For this review, take the finished solid that the model builds, in its own axes (mm). Face numbers are marked on the shaded views. A direction names the side the tool comes from. Give positions to 0.01 mm unless a question says otherwise; leave off trailing zeros. Loops run counter-clockwise (first coordinate to the right, second up) from the corner with the lowest first, then second, coordinate; pieces in that order, holes last. Notation, with made-up numbers: (82, 13) -> (116, 13) arc R28 ccw to (116, 34) -> close; hole circle Ø4 at (7.5, 22.25). An arc over 180 degrees is marked (long way). One line per question, with ' | ' between items. Start each with the question number.
(1) Insertion check: P1, Ø12, axis at x = 32.5, z = -18, coming from the -Y side; P2, Ø5, axis at x = -20.5, y = -17.5, coming from the -Z side; P3, Ø3, axis at x = 11, y = -30.5, coming from the -Z side; P4, Ø2, axis at y = -15.5, z = 0, coming from the -X side. Each pin has a flat end and moves straight along its axis. Give the tip position at first contact, or say it passes through.
(2) Consider section A-A (y = -17.5). Write out the cut boundary in (x, z), and give its area (3 significant figures).
(3) Consider section C-C (x = 27). Write out the cut boundary in (y, z), and give its area (3 significant figures).
(4) Tool access review of the marked faces 1, 2 and 3: name each direction out of +Z, -Z, +X, -X, +Y, -Y from which nothing blocks a thin tool from reaching the whole face with its end or side.
(5) Draft analysis for pull direction X (two halves, no side actions). For the marked faces 4, 5 and 6, state which applies: +X half, -X half, draft (parallel to the pull), parting line (faces both ways), or undercut.
(6) Consider section D-D (y = -6.5). Write out the cut boundary in (x, z).
(7) Wall thickness on probe 1 along X at (y, z) = (-6, 5); probe 2 along Z at (x, y) = (22, -32.5); probe 3 along Y at (x, z) = (-35, 7): over which ranges is each line inside the solid? List them lowest first.
(8) Consider section B-B (z = 0). Write out the cut boundary in (x, y), and give its area (3 significant figures).
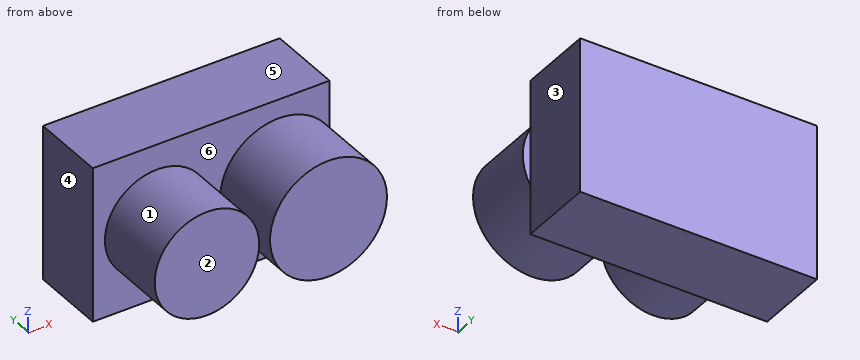
from build123d import *

# Parameters (mm, degrees)
F0_W     = 79.5864835382
F0_H     = 52.0435199142
F1_DEPTH = 12.7
F2_R     = 19.6570457416
F2_R_2   = 17.5585400789
F3_DEPTH = 25.4


with BuildPart() as f1:
    # F0 (on Front) → F1 (new body, symmetric)
    with BuildSketch(Plane.XZ):
        Rectangle(F0_W, F0_H)
    extrude(amount=F1_DEPTH, both=True)

    # F2 (on face) → F3 (join)
    with BuildSketch(Plane.XZ.offset(12.7)):
        with Locations((22.6829834282, 0)):
            Circle(F2_R)
        with Locations((-18.1834697723, 0)):
            Circle(F2_R_2)
    extrude(amount=F3_DEPTH)


solid = f1.part
A:
1) P1: stops at y = -38.1 | P2: stops at z = -17.56 | P3: stops at z = -16.81 | P4: stops at x = -35.74
2) outline: circle Ø35.12 at (-18.18, 0); circle Ø39.31 at (22.68, 0) | area: 2,180 mm^2
3) outline: (-38.1, -19.18) -> (-12.7, -19.18) -> (-12.7, -26.02) -> (12.7, -26.02) -> (12.7, 26.02) -> (-12.7, 26.02) -> (-12.7, 19.18) -> (-38.1, 19.18) -> close | area: 2,300 mm^2
4) face 1: -Y | face 2: +Z, -Z, +X, -X, -Y | face 3: +Z, -Z, +X, +Y
5) face 4: -X half | face 5: draft | face 6: undercut
6) outline: (-39.79, -26.02) -> (39.79, -26.02) -> (39.79, 26.02) -> (-39.79, 26.02) -> close
7) probe 1: x = -39.79 to 39.79 | probe 2: z = -19.65 to 19.65 | probe 3: y = -12.7 to 12.7
8) outline: (-39.79, -12.7) -> (-35.74, -12.7) -> (-35.74, -38.1) -> (-0.62, -38.1) -> (-0.62, -12.7) -> (3.03, -12.7) -> (3.03, -38.1) -> (42.34, -38.1) -> (42.34, -12.7) -> (39.79, -12.7) -> (39.79, 12.7) -> (-39.79, 12.7) -> close | area: 3,910 mm^2
